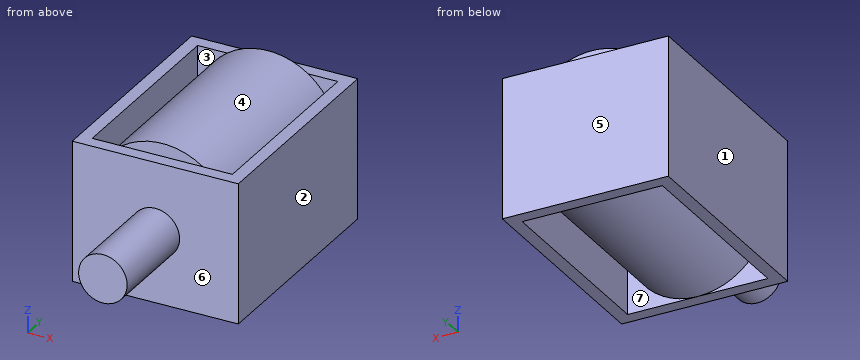
```python
from build123d import *

# Parameters (mm, degrees)
ESQUISSE1_W        = 15.4
ESQUISSE1_H        = 20.5
ESQUISSE1_W_2      = 13
ESQUISSE1_H_2      = 18.1
BOSS_EXTRU_1_DEPTH = 6.5
ESQUISSE2_R        = 2.25
BOSS_EXTRU_2_DEPTH = 9
BOSS_EXTRU_3_DEPTH = 18.1


with BuildPart() as part:
    # Esquisse1 → Boss.-Extru.1 (new, symmetric)
    with BuildSketch(Plane.XY):
        with Locations((0, 10.25)):
            Rectangle(ESQUISSE1_W, ESQUISSE1_H)
        with Locations((0, 10.25)):
            Rectangle(ESQUISSE1_W_2, ESQUISSE1_H_2, mode=Mode.SUBTRACT)
    extrude(amount=BOSS_EXTRU_1_DEPTH, both=True)

    # Esquisse2 → Boss.-Extru.2 (add)
    with BuildSketch(Plane.XZ):
        with Locations(Location((0, 0, 0), (0, 0, 90))):
            Circle(ESQUISSE2_R)
    extrude(amount=BOSS_EXTRU_2_DEPTH)

    # Esquisse3 → Boss.-Extru.3 (add)
    with BuildSketch(Plane(origin=(0, 1.2, 0), x_dir=(1, 0, 0), z_dir=(0, 1, 0))):
        with BuildLine():
            Line((6.5, 0), (6.5, -1.2))
            ThreePointArc((6.5, -1.2), (0, -7.7), (-6.5, -1.2))
            Line((-6.5, -1.2), (-6.5, 0))
            ThreePointArc((-6.5, 0), (0, 6.5), (6.5, 0))
        make_face()
    extrude(amount=BOSS_EXTRU_3_DEPTH)


solid = part.part
```
Verification items for the finished model (mm, model axes). Face numbers are marked on the shaded views. A direction names the side the tool comes from. Give positions to 0.01 mm unless a question says otherwise; leave off trailing zeros. Loops run counter-clockwise (first coordinate to the right, second up) from the corner with the lowest first, then second, coordinate; pieces in that order, holes last. Notation, with made-up numbers: M 19,20 L 63,20 A24 cw 63,43 Z; hole C 68,55 d2. An arc over 180 degrees is marked long. Return JSON: item names as keys, results as strings.
1) Section check C-C, the plane y = 6.75. Enter the section's corners in (x, z), and give its area (3 significant figures).
Findings:
{"outline": "M -7.7,-6.5 L -6.5,-6.5 L -6.5,0 A6.5 ccw 6.5,0 L 6.5,-6.5 L 7.7,-6.5 L 7.7,6.5 L 6.5,6.5 L 6.5,1.2 A6.5 ccw -6.5,1.2 L -6.5,6.5 L -7.7,6.5 Z", "area": "180 mm2"}
2) Mould release check, pull along X, two halves, no side actions. Record for the marked faces 1, 2, 3 and 4: released by +X, released by -X, zero draft, split by the parting line, or undercut.
Findings:
{"face 1": "released by -X", "face 2": "released by +X", "face 3": "undercut", "face 4": "undercut"}
3) Tool access check on the marked faces 5, 6 and 7. Record the directions out of +Z, -Z, +X, -X, +Y, -Y that give a thin tool (end or side, any length) a straight path to the whole face; none if there is none.
Findings:
{"face 5": "+Z, -Z, +X, -X, +Y", "face 6": "-Y", "face 7": "-Z"}
4) Gauge pin test, flat ends, axial feed: P1, Ø0.6, axis at x = 1, z = 7, coming from the -Y side; P2, Ø5, axis at x = 1.5, z = -5, coming from the -Y side; P3, Ø4, axis at x = -2.5, y = 10, coming from the -Z side; P4, Ø7.5, axis at x = 0.5, y = 6, coming from the +Z side. Record the tip position at first contact, or that the pin passes through.
Findings:
{"P1": "stops at y = 1.2", "P2": "stops at y = 0", "P3": "stops at z = -6.48", "P4": "stops at z = 7.7"}
5) Section check B-B, the plane x = -6. Enter the section's corners in (y, z).
Findings:
{"outline": "M 0,-6.5 L 1.2,-6.5 L 1.2,-2.5 L 19.3,-2.5 L 19.3,-6.5 L 20.5,-6.5 L 20.5,6.5 L 19.3,6.5 L 19.3,3.7 L 1.2,3.7 L 1.2,6.5 L 0,6.5 Z"}
6) Material ranges on L1, parallel to X at y = 7.75, z = -2.5; L2, parallel to X at y = 10.5, z = -3.5; L3, parallel to Z at x = -0.25, y = 17.25, recorded low to high. Write a range as [from, to].
Findings:
{"L1": "x = [-7.7, -6.5], [-6, 6], [6.5, 7.7]", "L2": "x = [-7.7, -6.5], [-5.48, 5.48], [6.5, 7.7]", "L3": "z = [-6.5, 7.7]"}
7) Section check A-A, the plane z = 4.5. Enter the section's corners in (x, y).
Findings:
{"outline": "M -7.7,0 L 7.7,0 L 7.7,20.5 L -7.7,20.5 Z; hole M -6.5,1.2 L -5.6,1.2 L -5.6,19.3 L -6.5,19.3 Z; hole M 5.6,1.2 L 6.5,1.2 L 6.5,19.3 L 5.6,19.3 Z"}
8) Section check D-D, the plane z = -1. Enter the section's corners in (x, y).
Findings:
{"outline": "M -7.7,0 L -2.02,0 L -2.02,-9 L 2.02,-9 L 2.02,0 L 7.7,0 L 7.7,20.5 L -7.7,20.5 Z; hole M -6.5,1.2 L -6.42,1.2 L -6.42,19.3 L -6.5,19.3 Z; hole M 6.42,1.2 L 6.5,1.2 L 6.5,19.3 L 6.42,19.3 Z"}
